from build123d import *

# Parameters (mm, degrees)
SKETCH1_W           = 51
SKETCH1_H           = 33
SKETCH1_W_2         = 47
SKETCH1_H_2         = 29
BOSS_EXTRUDE1_DEPTH = 50
SKETCH1_3_W         = 51
SKETCH1_3_H         = 33
SKETCH1_3_W_2       = 47
SKETCH1_3_H_2       = 29
SKETCH1_3_R         = 4.5
BOSS_EXTRUDE2_DEPTH = 5
SKETCH2_W           = 51
SKETCH2_H           = 3
BOSS_EXTRUDE3_DEPTH = 0.7


with BuildPart() as part:
    # Sketch1 → Boss-Extrude1 (new body)
    with BuildSketch(Plane.XY):
        Rectangle(SKETCH1_W, SKETCH1_H)
        Rectangle(SKETCH1_W_2, SKETCH1_H_2, mode=Mode.SUBTRACT)
    extrude(amount=BOSS_EXTRUDE1_DEPTH)

    # Sketch1_3 → Boss-Extrude2 (add)
    # profile 1 of 2: a face of its own
    with BuildSketch(Plane.XY):
        Rectangle(SKETCH1_3_W, SKETCH1_3_H)
        Rectangle(SKETCH1_3_W_2, SKETCH1_3_H_2, mode=Mode.SUBTRACT)
    # profile 2 of 2: a face of its own
    with BuildSketch(Plane.XY):
        Rectangle(SKETCH1_3_W_2, SKETCH1_3_H_2)
        Circle(SKETCH1_3_R, mode=Mode.SUBTRACT)
    extrude(amount=-BOSS_EXTRUDE2_DEPTH)

    # Sketch2 → Boss-Extrude3 (add)
    with BuildSketch(Plane.XY.offset(50)):
        with Locations((0, 15)):
            Rectangle(SKETCH2_W, SKETCH2_H)
        with Locations((0, -15)):
            Rectangle(SKETCH2_W, SKETCH2_H)
    extrude(amount=-BOSS_EXTRUDE3_DEPTH)


solid = part.part
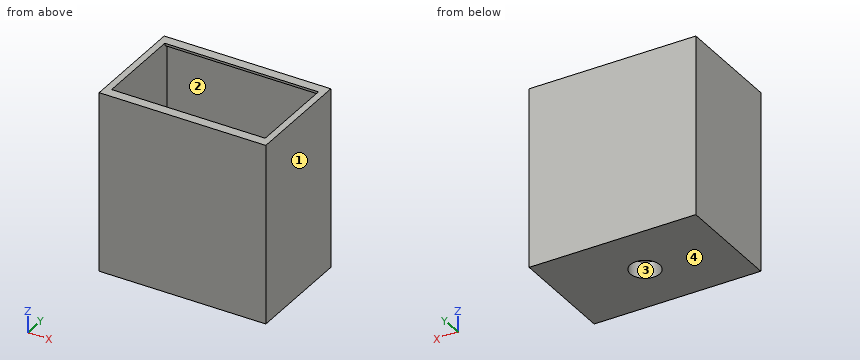
Source: CAD feature listing. Evaluate the final solid. Frame: model axes, mm. Face numbers are marked on the shaded views. Round coordinates to 2 decimals unless told otherwise and drop trailing zeros. Order: outer loops, then holes, each group sorted by start corner. A loop starts at its lowest first (then second) coordinate and runs counter-clockwise, first axis right, second up. Notation, with made-up numbers: (-34, 26.25) - (11, 26.25) arc R30 cw to (11, 56.25) - close; hole circle Ø1 at (9.25, 20.25). An arc over 180 degrees is marked (long way). Use a Markdown table: item, result. Add a question column.
1. Line query: probe 1 along X at (y, z) = (4.5, 31); probe 2 along Y at (x, z) = (8, 30.5); probe 3 along Y at (x, z) = (0, -3.85). Output: solid intervals per line, ascending.
2. First-contact query: pin 1 (10 mm diameter, centred on x = -5.5, y = -8, fed in from +Z). Flat tip, straight axial feed; report the tip coordinate or a pass-through.
3. Section query D-D (y = -8.5). Return the cut outline in (x, z).
4. Mould query, pull axis X, two halves, no side actions, for the marked faces 1, 2, 3 and 4. Classes: +X half, -X half, draft (parallel to the pull), parting line (faces both ways), or undercut.
5. Section query B-B (z = 18). Return the cut outline in (x, y).
6. Section query A-A (y = 0). Return the cut outline in (x, z), then the cut area to 3 significant figures.
7. Section query C-C (x = 0). Return the cut outline in (y, z).
Derived:
| question | item | result |
|---|---|---|
| 1 | probe 1 | -25.5 to -23.5, 23.5 to 25.5 |
| 1 | probe 2 | -16.5 to -14.5, 14.5 to 16.5 |
| 1 | probe 3 | -16.5 to -4.5, 4.5 to 16.5 |
| 2 | pin 1 | z = 0 |
| 3 | outline | (-25.5, -5) - (25.5, -5) - (25.5, 50) - (23.5, 50) - (23.5, 0) - (-23.5, 0) - (-23.5, 50) - (-25.5, 50) - close |
| 4 | face 1 | +X half |
| 4 | face 2 | undercut |
| 4 | face 3 | undercut |
| 4 | face 4 | draft |
| 5 | outline | (-25.5, -16.5) - (25.5, -16.5) - (25.5, 16.5) - (-25.5, 16.5) - close; hole (-23.5, -14.5) - (23.5, -14.5) - (23.5, 14.5) - (-23.5, 14.5) - close |
| 6 | outline | (-25.5, -5) - (-4.5, -5) - (-4.5, 0) - (-23.5, 0) - (-23.5, 50) - (-25.5, 50) - close; (4.5, -5) - (25.5, -5) - (25.5, 50) - (23.5, 50) - (23.5, 0) - (4.5, 0) - close |
| 6 | area | 410 mm2 |
| 7 | outline | (-16.5, -5) - (-4.5, -5) - (-4.5, 0) - (-14.5, 0) - (-14.5, 49.3) - (-13.5, 49.3) - (-13.5, 50) - (-16.5, 50) - close; (4.5, -5) - (16.5, -5) - (16.5, 50) - (13.5, 50) - (13.5, 49.3) - (14.5, 49.3) - (14.5, 0) - (4.5, 0) - close |
